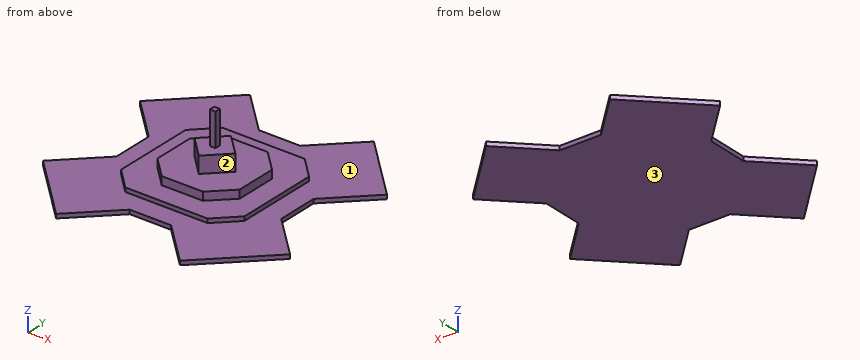
from build123d import *

# Parameters (mm, degrees)
F0_W     = 7.026562
F0_H     = 6.945758
F1_DEPTH = 81.28
F3_DEPTH = 40.64
F5_DEPTH = 20.32
F7_DEPTH = 10.16
F9_DEPTH = 5.08


with BuildPart() as f1:
    # F0 (on Top) → F1 (new body)
    with BuildSketch(Plane.XY):
        Rectangle(F0_W, F0_H)
    extrude(amount=F1_DEPTH)

    # F2 (on Top) → F3 (join)
    with BuildSketch(Plane.XY):
        Polygon((0, 25.393864), (-25.020789, 0), (0, -25.393864), (25.393864, 0), align=None)
    extrude(amount=F3_DEPTH)

    # F4 (on Top) → F5 (join)
    with BuildSketch(Plane.XY):
        Polygon((25.43629, 50.779495), (0, 50.779495), (-25.430322, 50.779495), (-50.833207, 25.546703), (-50.833207, 0), (-50.833207, -25.586797), (-25.600415, -50.989682), (25.266197, -50.819589), (50.669082, -25.586797), (50.669082, 25.37661), align=None)
    extrude(amount=F5_DEPTH)

    # F6 (on Top) → F7 (join)
    with BuildSketch(Plane.XY):
        Polygon((76.233596, -50.651934), (76.233596, 51.060922), (50.894871, 76.66897), (0, 76.66897), (-50.771996, 76.66897), (-76.126471, 51.060922), (-76.126471, -50.651934), (-50.771996, -76.197065), (0, -76.197065), (50.894871, -76.197065), align=None)
    extrude(amount=F7_DEPTH)

    # F8 (on Top) → F9 (join)
    with BuildSketch(Plane.XY):
        Polygon((-25.513835, -101.515338), (0, -101.515338), (25.52755, -101.515338), (76.299801, -152.375132), (152.654715, -76.282322), (101.746045, -25.306873), (101.746045, 25.734512), (152.605839, 76.506764), (76.51303, 152.861677), (25.53758, 101.953007), (-25.503805, 101.953007), (-76.276056, 152.812801), (-152.63097, 76.719992), (-101.7223, 25.744542), (-101.7223, -25.296843), (-152.582094, -76.069094), (-76.489285, -152.424008), align=None)
    extrude(amount=F9_DEPTH)


solid = f1.part
Read the model definition and answer for the solid it produces. Units are mm, in the model's axes. Face numbers are marked on the shaded views. Coordinates: 2 decimals unless noted, no trailing zeros. Order: outer loops, then holes, each group sorted by start corner. A loop starts at its lowest first (then second) coordinate and runs counter-clockwise, first axis right, second up. Notation, with made-up numbers: M 79.5,54.25 L 130.5,54.25 A17 cw 130.5,68.25 Z; hole C 65,-27.75 d6. An arc over 180 degrees is marked long. Put each result on its own line as item: value. Start each with the question number.
Item 1: Section A-A, the plane y = 119 is taken. Determine the outline of the cut face in (x, z), plus the area to 3 significant figures.
Item 2: Given pin 1 Ø11 at (y, z) = (1.5, 16.5) entering from -X; pin 2 Ø5.5 at (x, z) = (0, 66.5) entering from -Y; pin 3 Ø5.5 at (y, z) = (-1.5, 2.5) entering from -X, each flat-ended and moving along its own axis, determine where each tip first touches the part or whether it passes through.
Item 3: The mould has two halves that part along Z. Classify the marked faces 1, 2 and 3: +Z half, -Z half, draft (parallel to the pull), parting line (faces both ways), or undercut.
Item 4: Section C-C, the plane x = -30 is taken. Determine the outline of the cut face in (y, z), plus the area to 3 significant figures.
Item 5: Consider probe 1 along Y at (x, z) = (-14, 8); probe 2 along Z at (x, y) = (69, 34); probe 3 along Z at (x, y) = (19.5, 87.5). Determine where each line is inside the solid, lowest interval first. Write a range as [from, to].
Item 6: Section D-D, the plane y = 69.5 is taken. Determine the outline of the cut face in (x, z).
Item 7: Section B-B, the plane z = 16 is taken. Determine the outline of the cut face in (x, y), plus the area to 3 significant figures.
Computed:
1. outline: M -110.21,0 L -42.52,0 L -42.52,5.08 L -110.21,5.08 Z; M 42.61,0 L 110.26,0 L 110.26,5.08 L 42.61,5.08 Z
1. area: 688 mm2
2. pin 1: stops at x = -50.83
2. pin 2: stops at y = -3.47
2. pin 3: stops at x = -101.72
3. face 1: +Z half
3. face 2: draft
3. face 3: -Z half
4. outline: M -106,0 L 106.46,0 L 106.46,5.08 L 76.67,5.08 L 76.67,10.16 L 46.24,10.16 L 46.24,20.32 L -46.56,20.32 L -46.56,10.16 L -76.2,10.16 L -76.2,5.08 L -106,5.08 Z
4. area: 2,800 mm2
5. probe 1: y = [-76.2, 76.67]
5. probe 2: z = [0, 10.16]
5. probe 3: z = [0, 5.08]
6. outline: M -145.42,0 L 145.59,0 L 145.59,5.08 L 57.99,5.08 L 57.99,10.16 L -57.87,10.16 L -57.87,5.08 L -145.42,5.08 Z
7. outline: M -50.83,-25.59 L -25.6,-50.99 L 25.27,-50.82 L 50.67,-25.59 L 50.67,25.38 L 25.44,50.78 L -25.43,50.78 L -50.83,25.55 Z
7. area: 9,040 mm2
